The model under review builds one solid part; all positions refer to its coordinate system, in mm. A direction names the side the tool comes from. Coordinates: 2 decimals unless noted, no trailing zeros. Order: outer loops, then holes, each group sorted by start corner. A loop starts at its lowest first (then second) coordinate and runs counter-clockwise, first axis right, second up. Notation, with made-up numbers: M 20.25,49.25 L 49.25,49.25 A7 ccw 49.25,55.25 Z; hole C 16.5,-35 d7. An arc over 180 degrees is marked long. Write each question's results on one line, items separated by ' | '.
from build123d import *

# Parameters (mm, degrees)
F0_W     = 50.8
F0_H     = 38.1
F1_DEPTH = 31.75
F3_DEPTH = 31.75
F5_DEPTH = 19.05
F7_DEPTH = 12.7
F8_W     = 19.05
F8_H     = 25.4
F9_DEPTH = 19.05


with BuildPart() as f1:
    # F0 (on Right) → F1 (new body)
    with BuildSketch(Plane.YZ):
        with Locations((25.4, 19.05)):
            Rectangle(F0_W, F0_H)
    extrude(amount=F1_DEPTH)

    # F2 (on face) → F3 (cut)
    with BuildSketch(Plane.YZ.offset(31.75)):
        Polygon((50.8, 12.7), (50.8, 38.1), (38.1, 38.1), align=None)
    extrude(amount=-F3_DEPTH, mode=Mode.SUBTRACT)

    # F4 (on face) → F5 (cut)
    with BuildSketch(Plane.YZ.offset(31.75)):
        Polygon((31.75, 12.7), (50.8, 12.7), (38.1, 38.1), (31.75, 38.1), align=None)
    extrude(amount=-F5_DEPTH, mode=Mode.SUBTRACT)

    # F6 (on face) → F7 (cut)
    with BuildSketch(Plane(origin=(0, 31.75, 0), x_dir=(-1, 0, 0), z_dir=(0, 1, 0))):
        Polygon((-31.75, 38.1), (-31.75, 12.7), (-12.7, 38.1), align=None)
    extrude(amount=-F7_DEPTH, mode=Mode.SUBTRACT)

    # F8 (on face) → F9 (cut)
    with BuildSketch(Plane.YZ.offset(31.75)):
        with Locations((9.525, 25.4)):
            Rectangle(F8_W, F8_H)
    extrude(amount=-F9_DEPTH, mode=Mode.SUBTRACT)


solid = f1.part
1) Take a section at B-B on z = 26.5. State the section outline as (x, y) points, plus the area to 3 significant figures.
Solutions:
outline: M 0,0 L 12.7,0 L 12.7,19.05 L 21.4,19.05 L 21.4,31.75 L 12.7,31.75 L 12.7,43.9 L 0,43.9 Z | area: 668 mm2
2) Take a section at D-D on y = 8.5. State the section outline as (x, z) points, plus the area to 3 significant figures.
Solutions:
outline: M 0,0 L 31.75,0 L 31.75,12.7 L 12.7,12.7 L 12.7,38.1 L 0,38.1 Z | area: 726 mm2
3) To check wall thickness, follow line 1 along Y through (x, z) = (18, 28.5); line 2 along Z through (x, y) = (19.5, 16). State the ranges of each line that lie inside material, in increasing order.
Solutions:
line 1: 19.05 to 31.75 | line 2: 0 to 12.7
4) The part is to be moulded in two halves that separate along X. For faces 1 (the flat face through (18, 31.75, 20)), 2 (the flat face through (12.7, 9, 26)), 3 (the flat face through (0, 25, 19)), say which applies: pulls with the +X half, pulls with the -X half, needs draft (parallel to the pull), parting line crosses it, or undercut.
Solutions:
face 1: needs draft | face 2: pulls with the +X half | face 3: pulls with the -X half
5) Take a section at C-C on x = 16. State the section outline as (y, z) points, plus the area to 3 significant figures.
Solutions:
outline: M 0,0 L 50.8,0 L 50.8,12.7 L 31.75,12.7 L 31.75,33.7 L 19.05,33.7 L 19.05,12.7 L 0,12.7 Z | area: 912 mm2
6) Take a section at A-A on y = 40.5. State the section outline as (x, z) points.
Solutions:
outline: M 0,0 L 31.75,0 L 31.75,12.7 L 12.7,12.7 L 12.7,33.3 L 0,33.3 Z
7) For pin 1 (6 mm diameter, centred on x = 19.5, y = 19, fed in from +Z); pin 2 (15 mm diameter, centred on x = 23, z = 20.5, fed in from +Y); pin 3 (5.5 mm diameter, centred on x = 19.5, y = 5.5, fed in from +Z), all flat-tipped, find the tip position at first contact; note any pin that passes through.
Solutions:
pin 1: z = 33.03 | pin 2: y = 31.75 | pin 3: z = 12.7
8) For faces 4 (the flat face through (22, 9, 12.7)), 5 (the flat face through (16, 25, 0)), 6 (the flat face through (12.7, 39, 23)), list the 3-axis set-ups (+Z, -Z, +X, -X, +Y, -Y) from which the entire face can be reached by the end or side of a thin tool; tool diameter is ignored.
Solutions:
face 4: +Z, +X, -Y | face 5: -Z, +X, -X, +Y, -Y | face 6: +Z, +X, +Y
